Autodesk Inventor part; units mm, degrees
ref_plane "YZ Plane" through (0, 0, 0) normal (1, 0, 0) x (0, 1, 0)
ref_plane "XZ Plane" through (0, 0, 0) normal (0, 1, 0) x (-1, 0, 0)
ref_plane "XY Plane" through (0, 0, 0) normal (0, 0, 1) x (1, 0, 0)
sketch "Sketch1" plane through (0, 0, 0) normal (0, 0, 1) x (1, 0, 0)
  line L0 (0, 0) -> (150, 0)
  line L1 (150, 0) -> (150, 80)
  line L2 (150, 80) -> (0, 80)
  line L3 (0, 80) -> (0, 0)
  dimension "d0" = 150
  dimension "d1" = 80
extrude "Extrusion1" add sketch "Sketch1" along normal blind 5
sketch "Sketch2" plane through (0, 0, 5) normal (0, 0, 1) x (1, 0, 0)
  line L0 (0, 0) -> (150, 0)
  line L1 (150, 80) -> (0, 80)
  line L2 (129, 0) -> (21, 0)
  line L3 (21, 0) -> (21, 80)
  line L4 (21, 80) -> (129, 80)
  line L5 (129, 80) -> (129, 0)
  line L6 (126, 3) -> (24, 3)
  line L7 (24, 3) -> (24, 77)
  line L8 (24, 77) -> (126, 77)
  line L9 (126, 77) -> (126, 3)
  line L10 (150, 0) -> (150, 80)
  point P0 (129, 80)
  point P1 (21, 0)
  dimension "d4" = 108
  dimension "d5" = 102
  dimension "d6" = 3
  dimension "d7" = 3
  dimension "d8" = 3
  dimension "d9" = 21
extrude "Extrusion2" add sketch "Sketch2" along normal blind 20 contours L3 L1 L5 L0
chamfer "Chamfer1" distance 2 angle 45 1 edges at (75, 3, 25)
chamfer "Chamfer2" distance 2 angle 45 1 edges at (126, 40, 25)
chamfer "Chamfer3" distance 2 angle 45 2 edges at (75, 77, 25) (24, 40, 25)
sketch "Sketch3" plane through (0, 0, 5) normal (0, 0, 1) x (1, 0, 0)
  circle A0 centre (137.5, 15) radius 3.25
  circle A1 centre (137.5, 65) radius 3.25
  line L0 (150, 0) -> (150, 80)
  line L1 (129, 0) -> (150, 0)
  line L2 (75, -16.6248) -> (75, 70.7208)
  line L3 (0, 80) -> (0, 0)
  circle A2 centre (12.5, 15) radius 3.25
  circle A3 centre (12.5, 65) radius 3.25
  dimension "d21" = 6.5
  dimension "d22" = 6.5
  dimension "d23" = 12.5
  dimension "d24" = 12.5
  dimension "d25" = 50
  dimension "d26" = 15
  dimension "d27" = 75
extrude "Extrusion3" cut sketch "Sketch3" against normal blind 60
sketch "Sketch4" plane through (24, 3, 5) normal (0, 1, 0) x (1, 0, 0)
  line L0 (0, 0) -> (0, -18)
  line L1 (102, -18) -> (102, 10.1304)
  line L2 (102, 10.1304) -> (0, 10.1304)
  line L3 (0, 10.1304) -> (0, -18)
  line L4 (0, 0) -> (102, 0)
  line L5 (102, 0) -> (0, 0)
  line L6 (0, 0) -> (0, -34.2808)
  line L7 (0, -34.2808) -> (102, -34.2808)
  line L8 (102, -34.2808) -> (102, 0)
  point P0 (-24, 5)
extrude "Extrusion5" cut sketch "Sketch4" against normal blind 10 contours L4 L1 L8 L7 L6 L0
fillet "Fillet1" radius 2 1 edges at (127, 1, 25)
fillet "Fillet2" radius 1 3 edges at (126, 0.9369, 24.8478) (126, 0.0858, 25) (126, 2.2929, 23.7071)
properties part number "MediumHolder"
For this review, take the finished solid that the model builds, in its own axes (mm). A direction names the side the tool comes from. Round coordinates to 2 decimals unless told otherwise and drop trailing zeros. Write each loop counter-clockwise with the first axis right and the second up, starting at its lowest first coordinate (ties: lowest second). Pieces come first, ordered by that corner, then holes. Notation, with made-up numbers: M -14,51.25 L 21,51.25 A20 cw 21,80.25 Z; hole C 12,10.5 d1. An arc over 180 degrees is marked long. Write item = value, one per line. Start each with the question number.
(1) We need section C-C (z = 12). Give the boundary of the cut face in (x, y).
(2) We need section A-A (y = 65). Give the boundary of the cut face in (x, z), then the cut area to 3 significant figures.
(3) For faces 5 (the face through (75, 0, 2)), 6 (the face through (24, 39, 13)), 7 (the face through (139, 41, 5)), 8 (the face through (10, 41, 5)), 9 (the face through (12.077, 18.222, 2.535)), list the 3-axis set-ups (+Z, -Z, +X, -X, +Y, -Y) from which the entire face can be reached by the end or side of a thin tool; tool diameter is ignored.
(4) Clearance check with flat-ended pins moving along their axes: pin 1 Ø10 at (x, z) = (46, 14) entering from -Y; pin 2 Ø3 at (y, z) = (37.5, 18.5) entering from -X; pin 3 Ø2 at (x, y) = (29, 59.5) entering from +Z. State where each tip first meets the part, or that it passes through.
(5) We need section B-B (x = 12.5). Give the boundary of the cut face in (y, z), then the cut area to 3 significant figures.
(6) The part is to be moulded in two halves that separate along Y. For faces 1 (the face through (129, 41, 15)), 2 (the face through (140.6, 15.98, 2.54)), 3 (the face through (76, 80, 12)), 4 (the face through (11.795, 61.827, 2.535)), say which applies: +Y half, -Y half, draft (parallel to the pull), parting line (faces both ways), or undercut.
(7) We need section D-D (x = 56). Give the boundary of the cut face in (y, z).
(8) For line 1 along Y through (x, z) = (137.5, 3.8); line 2 along X through (y, z) = (10.5, 11); line 3 along Z through (x, y) = (35, 57), list the stretches that pass through material, from the lowest coordinate up.
Results found:
q1.outline = M 21,0 L 24,0 L 24,77 L 126,77 L 126,0 L 129,0 L 129,80 L 21,80 Z
q2.outline = M 0,0 L 9.25,0 L 9.25,5 L 0,5 Z; M 15.75,0 L 134.25,0 L 134.25,5 L 129,5 L 129,25 L 128,25 L 126,23 L 126,5 L 24,5 L 24,23 L 22,25 L 21,25 L 21,5 L 15.75,5 Z; M 140.75,0 L 150,0 L 150,5 L 140.75,5 Z
q2.area = 801 mm²
q3.face_5 = +Z, -Z, +X, -X, -Y
q3.face_6 = +Z, -Y
q3.face_7 = +Z, +X, +Y, -Y
q3.face_8 = +Z, -X, +Y, -Y
q3.face_9 = +Z, -Z
q4.pin_1 = 77
q4.pin_2 = 21
q4.pin_3 = 5
q5.outline = M 0,0 L 11.75,0 L 11.75,5 L 0,5 Z; M 18.25,0 L 61.75,0 L 61.75,5 L 18.25,5 Z; M 68.25,0 L 80,0 L 80,5 L 68.25,5 Z
q5.area = 335 mm²
q6.face_1 = draft
q6.face_2 = undercut
q6.face_3 = +Y half
q6.face_4 = undercut
q7.outline = M 0,0 L 80,0 L 80,25 L 79,25 L 77,23 L 77,5 L 0,5 Z
q8.line_1 = 0 to 11.75, 18.25 to 61.75, 68.25 to 80
q8.line_2 = 21 to 24, 126 to 129
q8.line_3 = 0 to 5
